```python
from build123d import *

# Parameters (mm, degrees)
SKETCH1_W                        = 58
SKETCH1_H                        = 44
BOSS_EXTRUDE1_DEPTH              = 11.5
F_16_5_16_5_DIAMETER_HOLE1_D     = 16.5
F_16_5_16_5_DIAMETER_HOLE1_DEPTH = 6
M3X0_5_TAPPED_HOLE1_D            = 2.5
M3X0_5_TAPPED_HOLE1_DEPTH        = 7.5
CUT_EXTRUDE1_DEPTH               = 10.3
CUT_EXTRUDE2_DEPTH               = 10.3
CUT_EXTRUDE3_DEPTH               = 39.173943993
M2_5X0_45_TAPPED_HOLE1_D         = 2.05
M2_5X0_45_TAPPED_HOLE1_DEPTH     = 6.35
SKETCH16_W                       = 13
SKETCH16_H                       = 4
CUT_EXTRUDE4_DEPTH               = 1.2


with BuildPart() as part:
    # Sketch1 → Boss-Extrude1 (new body)
    with BuildSketch(Plane(origin=(0, 0, 0), x_dir=(1, 0, 0), z_dir=(0, 1, 0))):
        Rectangle(SKETCH1_W, SKETCH1_H)
    extrude(amount=BOSS_EXTRUDE1_DEPTH)

    # 16.5 _16.5_ Diameter Hole1
    with Locations(Plane(origin=(0, 11.5, 0), x_dir=(1, 0, 0), z_dir=(0, 1, 0))):
        with Locations((0, 0)):
            Hole(F_16_5_16_5_DIAMETER_HOLE1_D / 2, depth=F_16_5_16_5_DIAMETER_HOLE1_DEPTH)

    # M3x0.5 Tapped Hole1
    with Locations(Plane(origin=(0, 11.5, 0), x_dir=(1, 0, 0), z_dir=(0, 1, 0))):
        with Locations((-10, 10), (10, 10), (-10, -10), (10, -10)):
            Hole(M3X0_5_TAPPED_HOLE1_D / 2, depth=M3X0_5_TAPPED_HOLE1_DEPTH)

    # Sketch10 → Cut-Extrude1 (cut)
    with BuildSketch(Plane.XZ):
        with BuildLine():
            ThreePointArc((-5.828427125, 16.5), (-5.956795679, 16.007305936), (-6, 15.5))
            ThreePointArc((-6, 15.5), (-5.121320344, 13.378679656), (-3, 12.5))
            Line((-3, 12.5), (3, 12.5))
            ThreePointArc((3, 12.5), (5.121320344, 13.378679656), (6, 15.5))
            ThreePointArc((6, 15.5), (5.956795679, 16.007305936), (5.828427125, 16.5))
            ThreePointArc((5.828427125, 16.5), (4.732050808, 15.050510257), (3, 14.5))
            Line((3, 14.5), (-3, 14.5))
            ThreePointArc((-3, 14.5), (-4.732050808, 15.050510257), (-5.828427125, 16.5))
        make_face()
        with BuildLine():
            ThreePointArc((-3, 18.5), (-4.732050808, 17.949489743), (-5.828427125, 16.5))
            ThreePointArc((-5.828427125, 16.5), (-4.732050808, 15.050510257), (-3, 14.5))
            Line((-3, 14.5), (3, 14.5))
            ThreePointArc((3, 14.5), (4.732050808, 15.050510257), (5.828427125, 16.5))
            ThreePointArc((5.828427125, 16.5), (4.732050808, 17.949489743), (3, 18.5))
            Line((3, 18.5), (-3, 18.5))
        make_face()
        with BuildLine():
            ThreePointArc((-5.828427125, 16.5), (-5.956795679, 16.992694064), (-6, 17.5))
            Line((-6, 17.5), (-6, 15.5))
            ThreePointArc((-6, 15.5), (-5.956795679, 16.007305936), (-5.828427125, 16.5))
        make_face()
        with BuildLine():
            Line((3, 20.5), (-3, 20.5))
            ThreePointArc((-3, 20.5), (-5.121320344, 19.621320344), (-6, 17.5))
            ThreePointArc((-6, 17.5), (-5.956795679, 16.992694064), (-5.828427125, 16.5))
            ThreePointArc((-5.828427125, 16.5), (-4.732050808, 17.949489743), (-3, 18.5))
            Line((-3, 18.5), (3, 18.5))
            ThreePointArc((3, 18.5), (4.732050808, 17.949489743), (5.828427125, 16.5))
            ThreePointArc((5.828427125, 16.5), (5.956795679, 16.992694064), (6, 17.5))
            ThreePointArc((6, 17.5), (5.121320344, 19.621320344), (3, 20.5))
        make_face()
        with BuildLine():
            Line((6, 15.5), (6, 17.5))
            ThreePointArc((6, 17.5), (5.956795679, 16.992694064), (5.828427125, 16.5))
            ThreePointArc((5.828427125, 16.5), (5.956795679, 16.007305936), (6, 15.5))
        make_face()
        with BuildLine():
            Line((6, -17.5), (6, -15.5))
            ThreePointArc((6, -15.5), (5.956795679, -16.007305936), (5.828427125, -16.5))
            ThreePointArc((5.828427125, -16.5), (5.956795679, -16.992694064), (6, -17.5))
        make_face()
        with BuildLine():
            ThreePointArc((-3, -12.5), (-5.121320344, -13.378679656), (-6, -15.5))
            ThreePointArc((-6, -15.5), (-5.956795679, -16.007305936), (-5.828427125, -16.5))
            ThreePointArc((-5.828427125, -16.5), (-4.732050808, -15.050510257), (-3, -14.5))
            Line((-3, -14.5), (3, -14.5))
            ThreePointArc((3, -14.5), (4.732050808, -15.050510257), (5.828427125, -16.5))
            ThreePointArc((5.828427125, -16.5), (5.956795679, -16.007305936), (6, -15.5))
            ThreePointArc((6, -15.5), (5.121320344, -13.378679656), (3, -12.5))
            Line((3, -12.5), (-3, -12.5))
        make_face()
        with BuildLine():
            ThreePointArc((-5.828427125, -16.5), (-5.956795674, -16.992694035), (-6, -17.499999942))
            ThreePointArc((-6, -17.499999942), (-5.121320364, -19.621320323), (-3, -20.5))
            Line((-3, -20.5), (3, -20.5))
            ThreePointArc((3, -20.5), (5.121320344, -19.621320344), (6, -17.5))
            ThreePointArc((6, -17.5), (5.956795679, -16.992694064), (5.828427125, -16.5))
            ThreePointArc((5.828427125, -16.5), (4.732050808, -17.949489743), (3, -18.5))
            Line((3, -18.5), (-3, -18.5))
            ThreePointArc((-3, -18.5), (-4.732050808, -17.949489743), (-5.828427125, -16.5))
        make_face()
        with BuildLine():
            ThreePointArc((-5.828427125, -16.5), (-5.956795679, -16.007305936), (-6, -15.5))
            Line((-6, -15.5), (-6, -17.499999942))
            ThreePointArc((-6, -17.499999942), (-5.956795674, -16.992694035), (-5.828427125, -16.5))
        make_face()
        with BuildLine():
            ThreePointArc((-3, -14.5), (-4.732050808, -15.050510257), (-5.828427125, -16.5))
            ThreePointArc((-5.828427125, -16.5), (-4.732050808, -17.949489743), (-3, -18.5))
            Line((-3, -18.5), (3, -18.5))
            ThreePointArc((3, -18.5), (4.732050808, -17.949489743), (5.828427125, -16.5))
            ThreePointArc((5.828427125, -16.5), (4.732050808, -15.050510257), (3, -14.5))
            Line((3, -14.5), (-3, -14.5))
        make_face()
    extrude(amount=-CUT_EXTRUDE1_DEPTH, mode=Mode.SUBTRACT)

    # Sketch11 → Cut-Extrude2 (cut)
    with BuildSketch(Plane.XZ):
        with BuildLine():
            ThreePointArc((-15, 4), (-15.251272405, 4.012659617), (-15.5, 4.050510257))
            ThreePointArc((-15.5, 4.050510257), (-15.748727595, 4.012659617), (-16, 4))
            Line((-16, 4), (-15, 4))
        make_face()
        with BuildLine():
            ThreePointArc((-15.5, 17.949489743), (-14.063508327, 17.08113883), (-13.5, 15.5))
            Line((-13.5, 15.5), (-13.5, 6.5))
            ThreePointArc((-13.5, 6.5), (-14.063508327, 4.91886117), (-15.5, 4.050510257))
            ThreePointArc((-15.5, 4.050510257), (-15.251272405, 4.012659617), (-15, 4))
            ThreePointArc((-15, 4), (-13.232233047, 4.732233047), (-12.5, 6.5))
            Line((-12.5, 6.5), (-12.5, 15.5))
            ThreePointArc((-12.5, 15.5), (-13.232233047, 17.267766953), (-15, 18))
            ThreePointArc((-15, 18), (-15.251272405, 17.987340383), (-15.5, 17.949489743))
        make_face()
        with BuildLine():
            ThreePointArc((-17.5, 15.5), (-16.936491673, 17.08113883), (-15.5, 17.949489743))
            ThreePointArc((-15.5, 17.949489743), (-15.748727595, 17.987340383), (-16, 18))
            ThreePointArc((-16, 18), (-17.767766953, 17.267766953), (-18.5, 15.5))
            Line((-18.5, 15.5), (-18.5, 6.5))
            ThreePointArc((-18.5, 6.5), (-17.767766953, 4.732233047), (-16, 4))
            ThreePointArc((-16, 4), (-15.748727595, 4.012659617), (-15.5, 4.050510257))
            ThreePointArc((-15.5, 4.050510257), (-16.936491673, 4.91886117), (-17.5, 6.5))
            Line((-17.5, 6.5), (-17.5, 15.5))
        make_face()
        with BuildLine():
            Line((-13.5, 6.5), (-13.5, 15.5))
            ThreePointArc((-13.5, 15.5), (-14.063508327, 17.08113883), (-15.5, 17.949489743))
            ThreePointArc((-15.5, 17.949489743), (-16.936491673, 17.08113883), (-17.5, 15.5))
            Line((-17.5, 15.5), (-17.5, 6.5))
            ThreePointArc((-17.5, 6.5), (-16.936491673, 4.91886117), (-15.5, 4.050510257))
            ThreePointArc((-15.5, 4.050510257), (-14.063508327, 4.91886117), (-13.5, 6.5))
        make_face()
        with BuildLine():
            ThreePointArc((-16, 18), (-15.748727595, 17.987340383), (-15.5, 17.949489743))
            ThreePointArc((-15.5, 17.949489743), (-15.251272405, 17.987340383), (-15, 18))
            Line((-15, 18), (-16, 18))
        make_face()
        with BuildLine():
            ThreePointArc((-16, -4), (-15.748727595, -4.012659617), (-15.5, -4.050510257))
            ThreePointArc((-15.5, -4.050510257), (-15.251272405, -4.012659617), (-15, -4))
            Line((-15, -4), (-16, -4))
        make_face()
        with BuildLine():
            ThreePointArc((-17.5, -6.5), (-16.936491673, -4.91886117), (-15.5, -4.050510257))
            ThreePointArc((-15.5, -4.050510257), (-15.748727595, -4.012659617), (-16, -4))
            ThreePointArc((-16, -4), (-17.767766953, -4.732233047), (-18.5, -6.5))
            Line((-18.5, -6.5), (-18.5, -15.5))
            ThreePointArc((-18.5, -15.5), (-17.767766953, -17.267766953), (-16, -18))
            ThreePointArc((-16, -18), (-15.748727595, -17.987340383), (-15.5, -17.949489743))
            ThreePointArc((-15.5, -17.949489743), (-16.936491673, -17.08113883), (-17.5, -15.5))
            Line((-17.5, -15.5), (-17.5, -6.5))
        make_face()
        with BuildLine():
            ThreePointArc((-15.5, -4.050510257), (-14.063508327, -4.91886117), (-13.5, -6.5))
            Line((-13.5, -6.5), (-13.5, -15.5))
            ThreePointArc((-13.5, -15.5), (-14.063508327, -17.08113883), (-15.5, -17.949489743))
            ThreePointArc((-15.5, -17.949489743), (-15.251272405, -17.987340383), (-15, -18))
            ThreePointArc((-15, -18), (-13.232233047, -17.267766953), (-12.5, -15.5))
            Line((-12.5, -15.5), (-12.5, -6.5))
            ThreePointArc((-12.5, -6.5), (-13.232233047, -4.732233047), (-15, -4))
            ThreePointArc((-15, -4), (-15.251272405, -4.012659617), (-15.5, -4.050510257))
        make_face()
        with BuildLine():
            Line((-13.5, -15.5), (-13.5, -6.5))
            ThreePointArc((-13.5, -6.5), (-14.063508327, -4.91886117), (-15.5, -4.050510257))
            ThreePointArc((-15.5, -4.050510257), (-16.936491673, -4.91886117), (-17.5, -6.5))
            Line((-17.5, -6.5), (-17.5, -15.5))
            ThreePointArc((-17.5, -15.5), (-16.936491673, -17.08113883), (-15.5, -17.949489743))
            ThreePointArc((-15.5, -17.949489743), (-14.063508327, -17.08113883), (-13.5, -15.5))
        make_face()
        with BuildLine():
            ThreePointArc((-15, -18), (-15.251272405, -17.987340383), (-15.5, -17.949489743))
            ThreePointArc((-15.5, -17.949489743), (-15.748727595, -17.987340383), (-16, -18))
            Line((-16, -18), (-15, -18))
        make_face()
    extrude(amount=-CUT_EXTRUDE2_DEPTH, mode=Mode.SUBTRACT)

    # Sketch13 → Cut-Extrude3 (cut, through all)
    with BuildSketch(Plane.XZ):
        with BuildLine():
            ThreePointArc((-26.25, 18), (-25.444543648, 19.944543648), (-23.5, 20.75))
            Line((-23.5, 20.75), (-29, 20.75))
            Line((-29, 20.75), (-29, -20.75))
            Line((-29, -20.75), (-23.5, -20.75))
            ThreePointArc((-23.5, -20.75), (-25.444543648, -19.944543648), (-26.25, -18))
            Line((-26.25, -18), (-26.25, 18))
        make_face()
        with BuildLine():
            ThreePointArc((-26.25, -18), (-23.5, -20.75), (-20.75, -18))
            Line((-20.75, -18), (-20.75, 18))
            ThreePointArc((-20.75, 18), (-23.5, 20.75), (-26.25, 18))
            Line((-26.25, 18), (-26.25, -18))
        make_face()
        with BuildLine():
            ThreePointArc((-23.5, 20.75), (-21.555456352, 19.944543648), (-20.75, 18))
            Line((-20.75, 18), (-20.75, 22))
            Line((-20.75, 22), (-29, 22))
            Line((-29, 22), (-29, 20.75))
            Line((-29, 20.75), (-23.5, 20.75))
        make_face()
        with BuildLine():
            Line((-20.75, -22), (-20.75, -18))
            ThreePointArc((-20.75, -18), (-21.555456352, -19.944543648), (-23.5, -20.75))
            Line((-23.5, -20.75), (-29, -20.75))
            Line((-29, -20.75), (-29, -22))
            Line((-29, -22), (-20.75, -22))
        make_face()
    extrude(amount=-CUT_EXTRUDE3_DEPTH, mode=Mode.SUBTRACT)

    # M2.5x0.45 Tapped Hole1
    with Locations(Plane(origin=(0, 0, 0), x_dir=(-1, 0, 0), z_dir=(0, -1, 0))):
        with Locations((-17.5, 6), (-17.5, -6), (-17.5, -18), (-17.5, 18)):
            Hole(M2_5X0_45_TAPPED_HOLE1_D / 2, depth=M2_5X0_45_TAPPED_HOLE1_DEPTH)

    # Sketch16 → Cut-Extrude4 (cut)
    with BuildSketch(Plane.XZ):
        with Locations((0, 16.5)):
            Rectangle(SKETCH16_W, SKETCH16_H)
    extrude(amount=-CUT_EXTRUDE4_DEPTH, mode=Mode.SUBTRACT)


solid = part.part
```
Verification items for the finished model (mm, model axes). A direction names the side the tool comes from. Coordinates: 2 decimals unless noted, no trailing zeros. Write each loop counter-clockwise with the first axis right and the second up, starting at its lowest first coordinate (ties: lowest second). Pieces come first, ordered by that corner, then holes. Notation, with made-up numbers: (22.5, -35) - (70.5, -35) arc R18 cw to (70.5, -13) - close; hole circle Ø2 at (6.25, 83.25). An arc over 180 degrees is marked (long way). Write item = value, one per line.
Q1. Cross-section at C-C (y = 9). Give the number of separate pieces and of enclosed holes in the cut face, plus the area to 3 significant figures.
Answer:
separate_pieces = 1
enclosed_holes = 9
area = 1,620 mm²
Q2. Access from +Z, -Z, +X, -X, +Y, -Y to the whole of each face (thin tool, end or side, straight path). Record for faces 5 (the face through (10, 4, 10)), 6 (the face through (4, 0, 0)), 7 (the face through (-6, 6, 17)).
Answer:
face_5 = +Y
face_6 = +Z, -Z, +X, -X, -Y
face_7 = -Y
Q3. Cross-section at A-A (x = 17.5). Enter the section's corners in (y, z) (3 decimals).
Answer:
outline = (0, -22) - (11.5, -22) - (11.5, 22) - (0, 22) - (0, 19.025) - (6.35, 19.025) - (6.35, 16.975) - (0, 16.975) - (0, 7.025) - (6.35, 7.025) - (6.35, 4.975) - (0, 4.975) - (0, -4.975) - (6.35, -4.975) - (6.35, -7.025) - (0, -7.025) - (0, -16.975) - (6.35, -16.975) - (6.35, -19.025) - (0, -19.025) - close
Q4. Material ranges on L1, parallel to X at y = 7, z = 14.5; L2, parallel to Z at x = 17.5, y = 1.5 (3 decimals); L3, parallel to X at y = 8.75, z = -10, recorded low to high. Write a range as from..to.
Answer:
L1 = -20.75..-18.5, -12.5..-5.83, 5.83..29
L2 = -22..-19.025, -16.975..-7.025, -4.975..4.975, 7.025..16.975, 19.025..22
L3 = -20.75..-18.5, -12.5..-11.25, -8.75..8.75, 11.25..29
Q5. Cross-section at D-D (x = 10.5). Enter the section's corners in (y, z), plus the area to 3 significant figures.
Answer:
outline = (0, -22) - (11.5, -22) - (11.5, -11.15) - (4, -11.15) - (4, -8.85) - (11.5, -8.85) - (11.5, 8.85) - (4, 8.85) - (4, 11.15) - (11.5, 11.15) - (11.5, 22) - (0, 22) - close
area = 472 mm²
Q6. Go/stop test with a flat-tipped pin: pin 1 Ø4 at (x, z) = (0.5, -15) entering from -Y. Record where the tip stops, or that it passes through.
Answer:
pin_1 = 10.3
Q7. Cross-section at B-B (z = -13.5). Enter the section's corners in (x, y).
Answer:
outline = (-20.75, 0) - (-18.5, 0) - (-18.5, 10.3) - (-12.5, 10.3) - (-12.5, 0) - (-5.24, 0) - (-5.24, 10.3) - (5.24, 10.3) - (5.24, 0) - (29, 0) - (29, 11.5) - (-20.75, 11.5) - close
Q8. Mould release check, pull along Z, two halves, no side actions. Record for faces 1 (the face through (29, 6, 0)), 2 (the face through (4, 6, 22)), 3 (the face through (17.367, 3.219, -19.016)), 4 (the face through (16.687, 3.219, 6.624)): released by +Z, released by -Z, zero draft, split by the parting line, or undercut.
Answer:
face_1 = zero draft
face_2 = released by +Z
face_3 = undercut
face_4 = undercut
